Input: dimensioned drawing with shaded views. Units: mm. Origin: part minimum x, y, z. A direction names the side the tool comes from. Give positions to 0.01 mm unless a question says otherwise; leave off trailing zeros. Write each loop counter-clockwise with the first axis right and the second up, starting at its lowest first coordinate (ties: lowest second). Pieces come first, ordered by that corner, then holes.
Q1. Mould query, pull axis X, two halves, no side actions, for the marked faces 1, 2 and 3. Classes: +X half, -X half, draft (parallel to the pull), parting line (faces both ways), or undercut.
Q2. Line query: line 1 (Y direction, x = 14, z = 0.7); line 2 (X direction, y = 2.25, z = 0.45); line 3 (Z direction, x = 0.5, y = 12). Output: solid intervals per line, ascending.
Q3. Section D-D (y = 2.75). Return the cut outline in (x, z), plus the area to 3 significant figures.
Q4. Section A-A (x = 10). Return the cut outline in (y, z).
Q5. Section C-C (x = 14). Return the cut outline in (y, z), plus the area to 3 significant figures.
Q6. Section B-B (z = 2.6). Return the cut outline in (x, y).
Q7. Pin query (flat end, axial travel): pin 1 Ø1 at (y, z) = (12, 4.5) entering from -X; pin 2 Ø0.9 at (x, z) = (8, 1) entering from -Y; pin 3 Ø3 at (x, y) = (3, 16) entering from +Z. Return the tip coordinate at first contact, or that it passes through.
Q8. Reachability of the marked faces 4, 5, 6, 7 and 8 from +Z, -Z, +X, -X, +Y, -Y: full face, straight path, thin tool, end or side. Return the list, or none.
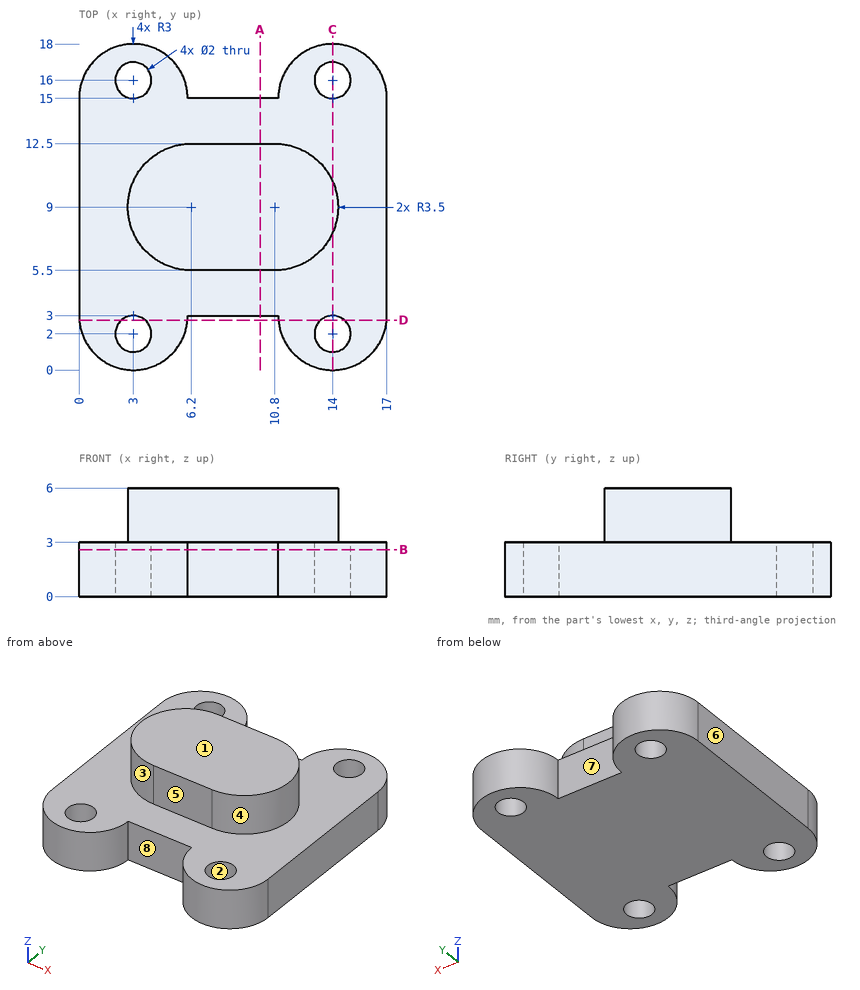
Computed:
1. face 1: draft
1. face 2: undercut
1. face 3: -X half
2. line 1: y = 0 to 1, 3 to 15, 17 to 18
2. line 2: x = 0.1 to 2.03, 3.97 to 5.9, 11.1 to 13.03, 14.97 to 16.9
2. line 3: z = 0 to 3
3. outline: (0.01, 0) - (2.34, 0) - (2.34, 3) - (0.01, 3) - close; (3.66, 0) - (5.99, 0) - (5.99, 3) - (3.66, 3) - close; (11.01, 0) - (13.34, 0) - (13.34, 3) - (11.01, 3) - close; (14.66, 0) - (16.99, 0) - (16.99, 3) - (14.66, 3) - close
3. area: 27.9 mm2
4. outline: (3, 0) - (15, 0) - (15, 3) - (12.5, 3) - (12.5, 6) - (5.5, 6) - (5.5, 3) - (3, 3) - close
5. outline: (0, 0) - (1, 0) - (1, 3) - (0, 3) - close; (3, 0) - (15, 0) - (15, 3) - (10.42, 3) - (10.42, 6) - (7.58, 6) - (7.58, 3) - (3, 3) - close; (17, 0) - (18, 0) - (18, 3) - (17, 3) - close
5. area: 50.5 mm2
6. outline: (0, 3) arc R3 ccw to (6, 3) - (11, 3) arc R3 ccw to (17, 3) - (17, 15) arc R3 ccw to (11, 15) - (6, 15) arc R3 ccw to (0, 15) - close; hole circle Ø2 at (3, 2); hole circle Ø2 at (3, 16); hole circle Ø2 at (14, 2); hole circle Ø2 at (14, 16)
7. pin 1: stops at x = 3.75
7. pin 2: stops at y = 3
7. pin 3: stops at z = 3
8. face 4: +Z, +X
8. face 5: +Z, +X, -X, -Y
8. face 6: +Z, -Z, -X, +Y, -Y
8. face 7: +Z, -Z, +Y
8. face 8: +Z, -Z, -Y
